For this review, take the finished solid that the model builds, in its own axes (mm). Give positions to 0.01 mm unless a question says otherwise; leave off trailing zeros. Write each loop counter-clockwise with the first axis right and the second up, starting at its lowest first coordinate (ties: lowest second). Pieces come first, ordered by that corner, then holes.
Q1. Insertion check: P1, Ø3, axis at x = 254.6, y = 35, coming from the +Z side. The pin has a flat end and moves straight along its axis. Give the tip position at first contact, or say it passes through.
Q2. For line 1 (Y direction, x = 139.1, z = 2.35); line 2 (X direction, y = 141, z = 1.95); line 3 (X direction, y = 59.5, z = 2.1), list the stretches that pass through material, from the lowest coordinate up.
Q3. We need section A-A (x = 139.1). Write out the cut boundary in (y, z), then the cut area to 3 significant figures.
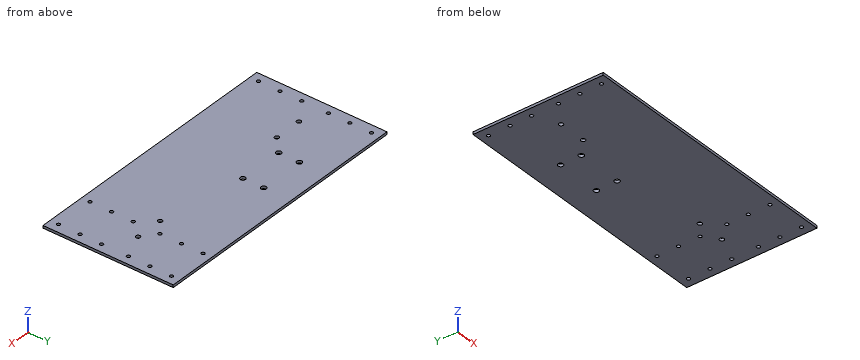
```python
from build123d import *

# Parameters (mm, degrees)
SKIZZE1_W                       = 310.4
SKIZZE1_H                       = 151
AUFSATZ_LINEAR_AUSTRAGEN1_DEPTH = 3
SKIZZE2_R                       = 2
SCHNITT_LINEAR_AUSTRAGEN1_DEPTH = 10
SKIZZE3_R                       = 2
SCHNITT_LINEAR_AUSTRAGEN2_DEPTH = 10
SKIZZE4_R                       = 3
SCHNITT_LINEAR_AUSTRAGEN3_DEPTH = 10
SKIZZE5_R                       = 2.5
SCHNITT_LINEAR_AUSTRAGEN4_DEPTH = 10
SKIZZE6_R                       = 2.5
SCHNITT_LINEAR_AUSTRAGEN5_DEPTH = 10


with BuildPart() as part:
    # Skizze1 → Aufsatz-Linear austragen1 (new body)
    with BuildSketch(Plane.XY):
        with Locations((155.2, 75.5)):
            Rectangle(SKIZZE1_W, SKIZZE1_H)
    extrude(amount=AUFSATZ_LINEAR_AUSTRAGEN1_DEPTH)

    # Skizze2 → Schnitt-Linear austragen1 (cut)
    with BuildSketch(Plane(origin=(0, 0, 0), x_dir=(-1, 0, 0), z_dir=(0, 0, -1))):
        with Locations((-300.4, 116)):
            Circle(SKIZZE2_R)
        with Locations((-300.4, 141)):
            Circle(SKIZZE2_R)
        with Locations((-300.4, 60)):
            Circle(SKIZZE2_R)
        with Locations((-300.4, 91)):
            Circle(SKIZZE2_R)
        with Locations((-300.4, 35)):
            Circle(SKIZZE2_R)
        with Locations((-300.4, 10)):
            Circle(SKIZZE2_R)
        with Locations((-10, 141)):
            Circle(SKIZZE2_R)
        with Locations((-10, 116)):
            Circle(SKIZZE2_R)
        with Locations((-10, 91)):
            Circle(SKIZZE2_R)
        with Locations((-10, 60)):
            Circle(SKIZZE2_R)
        with Locations((-10, 35)):
            Circle(SKIZZE2_R)
        with Locations((-10, 10)):
            Circle(SKIZZE2_R)
    extrude(amount=-SCHNITT_LINEAR_AUSTRAGEN1_DEPTH, mode=Mode.SUBTRACT)

    # Skizze3 → Schnitt-Linear austragen2 (cut)
    with BuildSketch(Plane(origin=(0, 0, 0), x_dir=(-1, 0, 0), z_dir=(0, 0, -1))):
        with Locations((-254.6, 10)):
            Circle(SKIZZE3_R)
        with Locations((-254.6, 35)):
            Circle(SKIZZE3_R)
        with Locations((-254.6, 60)):
            Circle(SKIZZE3_R)
        with Locations((-254.6, 91)):
            Circle(SKIZZE3_R)
        with Locations((-254.6, 116)):
            Circle(SKIZZE3_R)
        with Locations((-254.6, 141)):
            Circle(SKIZZE3_R)
    extrude(amount=-SCHNITT_LINEAR_AUSTRAGEN2_DEPTH, mode=Mode.SUBTRACT)

    # Skizze4 → Schnitt-Linear austragen3 (cut)
    with BuildSketch(Plane(origin=(0, 0, 0), x_dir=(-1, 0, 0), z_dir=(0, 0, -1))):
        with Locations((-139.1, 119)):
            Circle(SKIZZE4_R)
        with Locations((-87.1, 119)):
            Circle(SKIZZE4_R)
        with Locations((-139.1, 95)):
            Circle(SKIZZE4_R)
        with Locations((-87.1, 95)):
            Circle(SKIZZE4_R)
    extrude(amount=-SCHNITT_LINEAR_AUSTRAGEN3_DEPTH, mode=Mode.SUBTRACT)

    # Skizze5 → Schnitt-Linear austragen4 (cut)
    with BuildSketch(Plane(origin=(0, 0, 0), x_dir=(-1, 0, 0), z_dir=(0, 0, -1))):
        with Locations((-270.6, 78.5)):
            Circle(SKIZZE5_R)
        with Locations((-238.6, 78.5)):
            Circle(SKIZZE5_R)
    extrude(amount=-SCHNITT_LINEAR_AUSTRAGEN4_DEPTH, mode=Mode.SUBTRACT)

    # Skizze6 → Schnitt-Linear austragen5 (cut)
    with BuildSketch(Plane(origin=(0, 0, 0), x_dir=(-1, 0, 0), z_dir=(0, 0, -1))):
        with Locations((-69.1, 78.5)):
            Circle(SKIZZE6_R)
        with Locations((-37.1, 78.5)):
            Circle(SKIZZE6_R)
    extrude(amount=-SCHNITT_LINEAR_AUSTRAGEN5_DEPTH, mode=Mode.SUBTRACT)


solid = part.part
```
Computed:
1. P1: passes through
2. line 1: y = 0 to 92, 98 to 116, 122 to 151
2. line 2: x = 0 to 8, 12 to 252.6, 256.6 to 298.4, 302.4 to 310.4
2. line 3: x = 0 to 8.06, 11.94 to 252.66, 256.54 to 298.46, 302.34 to 310.4
3. outline: (0, 0) - (92, 0) - (92, 3) - (0, 3) - close; (98, 0) - (116, 0) - (116, 3) - (98, 3) - close; (122, 0) - (151, 0) - (151, 3) - (122, 3) - close
3. area: 417 mm2
